```python
from build123d import *

# Parameters (mm, degrees)
SKETCH1_R           = 1.143
SKETCH1_R_2         = 0.508
SKETCH1_R_3         = 1.0922
BOSS_EXTRUDE1_DEPTH = 0.8255
SKETCH2_W           = 7.62
SKETCH2_H           = 5.588
BOSS_EXTRUDE2_DEPTH = 2.54
SKETCH3_W           = 5.334
SKETCH3_H           = 5.334
BOSS_EXTRUDE3_DEPTH = 0.635


with BuildPart() as part:
    # Sketch1 → Boss-Extrude1 (new body)
    with BuildSketch(Plane.XY):
        Polygon((0, 26.67), (15.24, 26.67), (15.24, 3.048), (13.97, 1.778), (11.811, 1.778), (10.033, 0), (3.048, 0), (1.27, 1.778), (0, 1.778), align=None)
        with Locations(Location((1.905, 3.81, 0), (0, 0, 180))):
            Circle(SKETCH1_R, mode=Mode.SUBTRACT)
        with Locations(Location((13.335, 3.81, 0), (0, 0, 180))):
            Circle(SKETCH1_R, mode=Mode.SUBTRACT)
        with Locations((1.27, 6.858)):
            Circle(SKETCH1_R_2, mode=Mode.SUBTRACT)
        with Locations((1.27, 9.398)):
            Circle(SKETCH1_R_2, mode=Mode.SUBTRACT)
        with Locations((1.27, 11.938)):
            Circle(SKETCH1_R_2, mode=Mode.SUBTRACT)
        with Locations((1.27, 14.478)):
            Circle(SKETCH1_R_2, mode=Mode.SUBTRACT)
        with Locations((1.27, 17.018)):
            Circle(SKETCH1_R_2, mode=Mode.SUBTRACT)
        with Locations((13.97, 17.018)):
            Circle(SKETCH1_R_2, mode=Mode.SUBTRACT)
        with Locations((13.97, 14.478)):
            Circle(SKETCH1_R_2, mode=Mode.SUBTRACT)
        with Locations((13.97, 11.938)):
            Circle(SKETCH1_R_2, mode=Mode.SUBTRACT)
        with Locations((13.97, 9.398)):
            Circle(SKETCH1_R_2, mode=Mode.SUBTRACT)
        with Locations((13.97, 6.858)):
            Circle(SKETCH1_R_2, mode=Mode.SUBTRACT)
        with Locations(Location((1.524, 20.066, 0), (0, 0, 180))):
            Circle(SKETCH1_R_3, mode=Mode.SUBTRACT)
        with Locations(Location((13.716, 20.066, 0), (0, 0, 180))):
            Circle(SKETCH1_R_3, mode=Mode.SUBTRACT)
    extrude(amount=BOSS_EXTRUDE1_DEPTH)

    # Sketch2 → Boss-Extrude2 (add)
    with BuildSketch(Plane.XY.offset(0.8255)):
        with Locations((7.62, 24.638)):
            Rectangle(SKETCH2_W, SKETCH2_H)
    extrude(amount=BOSS_EXTRUDE2_DEPTH)

    # Sketch3 → Boss-Extrude3 (add)
    with BuildSketch(Plane.XY.offset(0.8255)):
        with Locations((8.255, 18.161)):
            Rectangle(SKETCH3_W, SKETCH3_H)
    extrude(amount=BOSS_EXTRUDE3_DEPTH)


solid = part.part
```
Part model, mm, in its own coordinate system. Round coordinates to 2 decimals unless told otherwise and drop trailing zeros. Write each loop counter-clockwise with the first axis right and the second up, starting at its lowest first coordinate (ties: lowest second). Pieces come first, ordered by that corner, then holes. Notation, with made-up numbers: (38.25, -10.75) -> (64.25, -10.75) arc R29 cw to (64.25, 17.25) -> close; hole circle Ø5 at (72, 58.5). An arc over 180 degrees is marked (long way). Return JSON: item names as keys, results as strings. Group by question number.
Q1. Mould opens along X. For faces 1 (the cylindrical face through (2.054, 2.677, 0.407)), 2 (the flat face through (11.43, 25, 2)), 3 (the flat face through (7.5, 26.67, 0.4)) say: pulls with the +X half, pulls with the -X half, needs draft (parallel to the pull), parting line crosses it, or undercut.
Q2. Probe L1, parallel to X at y = 20, z = 0.2; L2, parallel to X at y = 14.75, z = 0.2; L3, parallel to Z at x = 11.5, y = 14. List the from-to ranges inside material, lowest first. Write a range as [from, to].
Q3. Saw through at A-A on y = 3.81. Write the cut outline in (x, z).
Q4. Saw through at D-D on z = 0.5. State how many separate pieces and enclosed holes the cut face has, plus the area to 3 significant figures.
Q5. Saw through at B-B on y = 25.25. Write the cut outline in (x, z).
Q6. Pin check, flat tips, straight feed: pin 1 (1 mm diameter, centred on x = 11.5, z = 1, fed in from +Y); pin 2 (2 mm diameter, centred on x = 2, y = 4, fed in from +Z); pin 3 (0.7 mm diameter, centred on x = 12.5, z = 0.5, fed in from -Y); pin 4 (1.5 mm diameter, centred on x = 6.5, y = 19.5, fed in from +Z). Stop position of each tip, or through.
Q7. Saw through at C-C on x = 6.25. Write the cut outline in (y, z).
Answer:
{
 "1": {"face 1": "undercut", "face 2": "pulls with the +X half", "face 3": "needs draft"},
 "2": {"L1": "[0, 0.43], [2.61, 12.63], [14.81, 15.24]", "L2": "[0, 0.84], [1.7, 13.54], [14.4, 15.24]", "L3": "[0, 0.83]"},
 "3": {"outline": "(0, 0) -> (0.76, 0) -> (0.76, 0.83) -> (0, 0.83) -> close; (3.05, 0) -> (12.19, 0) -> (12.19, 0.83) -> (3.05, 0.83) -> close; (14.48, 0) -> (15.24, 0) -> (15.24, 0.83) -> (14.48, 0.83) -> close"},
 "4": {"separate pieces": "1", "enclosed holes": "14", "area": "370 mm2"},
 "5": {"outline": "(0, 0) -> (15.24, 0) -> (15.24, 0.83) -> (11.43, 0.83) -> (11.43, 3.37) -> (3.81, 3.37) -> (3.81, 0.83) -> (0, 0.83) -> close"},
 "6": {"pin 1": "y = 27.43", "pin 2": "z = 0.83", "pin 3": "y = 1.78", "pin 4": "z = 1.46"},
 "7": {"outline": "(0, 0) -> (26.67, 0) -> (26.67, 0.83) -> (27.43, 0.83) -> (27.43, 3.37) -> (21.84, 3.37) -> (21.84, 0.83) -> (20.83, 0.83) -> (20.83, 1.46) -> (15.49, 1.46) -> (15.49, 0.83) -> (0, 0.83) -> close"}
}
